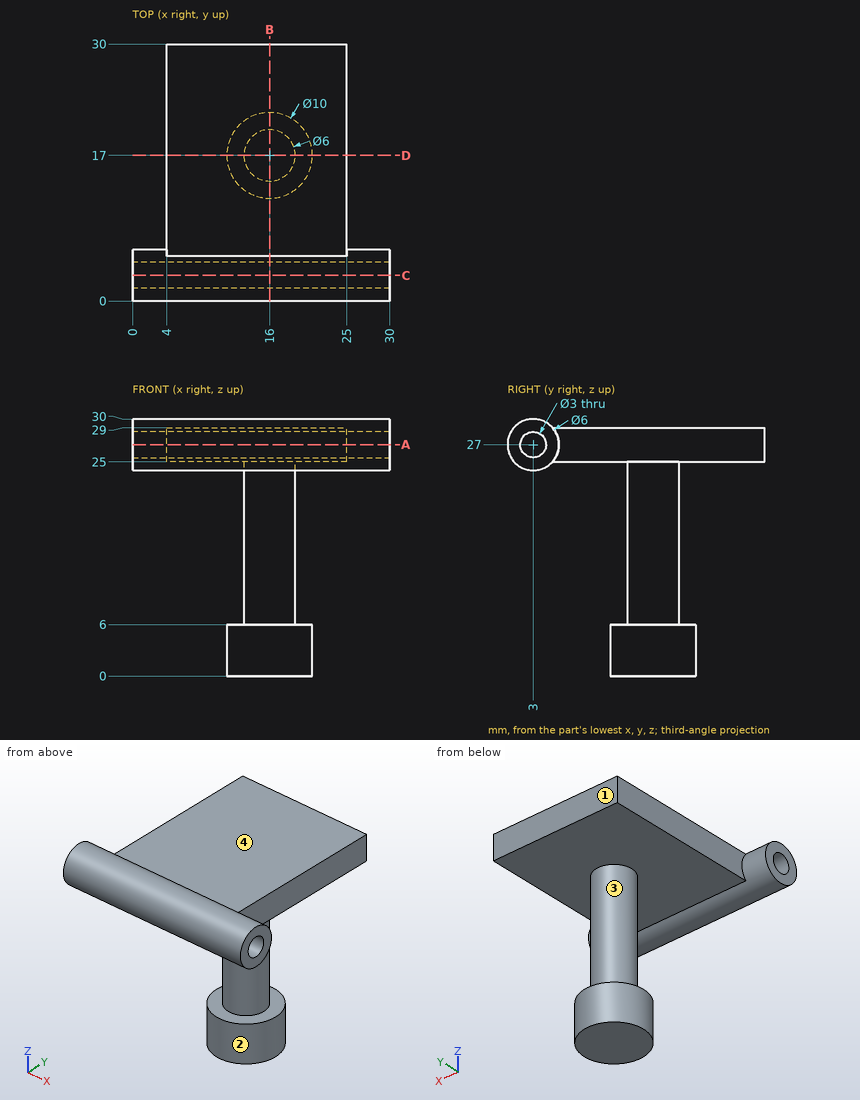
Verification items for this drawing (mm, ordinates from the low corner). A direction names the side the tool comes from. Round coordinates to 2 decimals unless told otherwise and drop trailing zeros. Order: outer loops, then holes, each group sorted by start corner. A loop starts at its lowest first (then second) coordinate and runs counter-clockwise, first axis right, second up.
1) Cross-section at C-C, the plane y = 3. Record the cut outline in (x, z), plus the area to 3 significant figures.
Geometry says:
outline: (0, 24) - (30, 24) - (30, 25.5) - (0, 25.5) - close; (0, 28.5) - (30, 28.5) - (30, 30) - (0, 30) - close
area: 90.0 mm2
2) Tool access check on the marked faces 1, 2, 3 and 4. Record the directions out of +Z, -Z, +X, -X, +Y, -Y that give a thin tool (end or side, any length) a straight path to the whole face; none if there is none.
Geometry says:
face 1: +Z, -Z, +X, -X, +Y
face 2: -Z
face 3: none
face 4: +Z, +X, -X, +Y
3) Cross-section at B-B, the plane x = 16. Record the cut outline in (y, z).
Geometry says:
outline: (5.24, 25) - (14, 25) - (14, 6) - (12, 6) - (12, 0) - (22, 0) - (22, 6) - (20, 6) - (20, 25) - (30, 25) - (30, 29) - (5.24, 29) arc R3 ccw (long way) to start; hole circle Ø3 at (3, 27)
4) Cross-section at D-D, the plane y = 17. Record the cut outline in (x, z), plus the area to 3 significant figures.
Geometry says:
outline: (4, 25) - (13, 25) - (13, 6) - (11, 6) - (11, 0) - (21, 0) - (21, 6) - (19, 6) - (19, 25) - (25, 25) - (25, 29) - (4, 29) - close
area: 258 mm2
5) Material ranges on line 1 (Y direction, x = 7.5, z = 27); line 2 (Z direction, x = 4.25, y = 6.25); line 3 (X direction, y = 21, z = 28.75), recorded low to high.
Geometry says:
line 1: y = 0 to 1.5, 4.5 to 30
line 2: z = 25 to 29
line 3: x = 4 to 25
6) Depth check by flat-ended pin: pin 1 (2 mm diameter, centred on y = 14, z = 26.5, fed in from +X); pin 2 (8 mm diameter, centred on x = 27, y = 9.5, fed in from +Z); pin 3 (1 mm diameter, centred on y = 15.5, z = 15.5, fed in from -X); pin 4 (10.5 mm diameter, centred on x = 14.5, y = 15.5, fed in from -Z). Enter the tip coordinate at first touch or a pass-through.
Geometry says:
pin 1: stops at x = 25
pin 2: stops at z = 29
pin 3: stops at x = 13.17
pin 4: stops at z = 0
7) Cross-section at A-A, the plane z = 27. Record the cut outline in (x, y), plus the area to 3 significant figures.
Geometry says:
outline: (0, 0) - (30, 0) - (30, 1.5) - (0, 1.5) - close; (0, 4.5) - (30, 4.5) - (30, 6) - (25, 6) - (25, 30) - (4, 30) - (4, 6) - (0, 6) - close
area: 594 mm2
